Source: CAD feature listing. Evaluate the final solid. Frame: model axes, mm. Face numbers are marked on the shaded views. Give positions to 0.01 mm unless a question says otherwise; leave off trailing zeros. Loops run counter-clockwise (first coordinate to the right, second up) from the corner with the lowest first, then second, coordinate; pieces in that order, holes last. Notation, with made-up numbers: M 69,-17 L 89,-17 A13 ccw 89,-12 Z; hole C -26.5,0 d7. An arc over 180 degrees is marked long. Put each result on its own line as item: value. Start each with the question number.
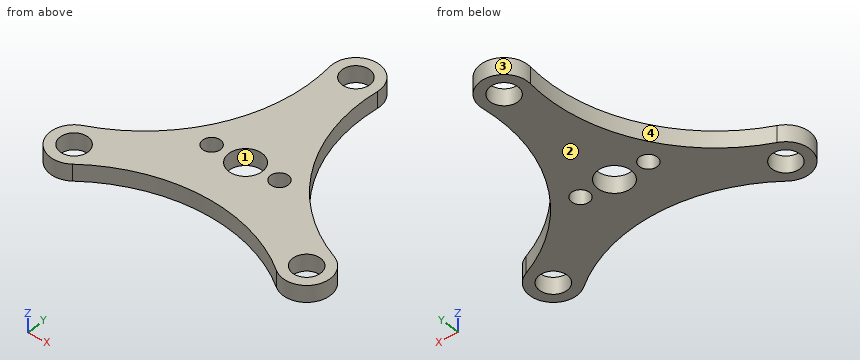
```python
from build123d import *

# Parameters (mm, degrees)
SKETCH_1_R      = 2.5
SKETCH_1_R_2    = 3
SKETCH_1_R_3    = 1.6
EXTRUDE_1_DEPTH = 3


with BuildPart() as part:
    # ｽｹｯﾁ1 → ﾎﾞｽ - 押し出し1 (new body)
    with BuildSketch(Plane.XY):
        with BuildLine():
            ThreePointArc((-22.235006429, -7.965532761), (-24.248711306, -14), (-18.01585694, -15.27331404))
            ThreePointArc((-18.01585694, -15.27331404), (0, -9.261413146), (18.01585694, -15.27331404))
            ThreePointArc((18.01585694, -15.27331404), (24.248711306, -14), (22.235006429, -7.965532761))
            ThreePointArc((22.235006429, -7.965532761), (8.020619059, 4.630706573), (4.219149489, 23.238846801))
            ThreePointArc((4.219149489, 23.238846801), (0, 28), (-4.219149489, 23.238846801))
            ThreePointArc((-4.219149489, 23.238846801), (-8.020619059, 4.630706573), (-22.235006429, -7.965532761))
        make_face()
        with Locations((0, 23.75)):
            Circle(SKETCH_1_R, mode=Mode.SUBTRACT)
        Circle(SKETCH_1_R_2, mode=Mode.SUBTRACT)
        with Locations((-6, 0)):
            Circle(SKETCH_1_R_3, mode=Mode.SUBTRACT)
        with Locations((6, 0)):
            Circle(SKETCH_1_R_3, mode=Mode.SUBTRACT)
        with Locations((20.56810334, -11.875)):
            Circle(SKETCH_1_R, mode=Mode.SUBTRACT)
        with Locations((-20.56810334, -11.875)):
            Circle(SKETCH_1_R, mode=Mode.SUBTRACT)
    extrude(amount=EXTRUDE_1_DEPTH)


solid = part.part
```
1. Pull-direction query (X, two-part tool) for the marked faces 1, 2, 3 and 4; classes: released by +X, released by -X, zero draft, split by the parting line, or undercut.
2. Section A-A, the plane x = 0. Output: boundary loops of the cut face in (y, z), plus the area to 3 significant figures.
3. Section C-C, the plane z = 1.3. Output: boundary loops of the cut face in (x, y) (3 decimals), plus the area to 3 significant figures.
4. Section D-D, the plane y = 0. Output: boundary loops of the cut face in (x, z), plus the area to 3 significant figures.
5. Ray query, line 1 (Y direction, x = 0, z = 2.3); line 2 (X direction, y = -14, z = 2.65); line 3 (Y direction, x = -22, z = 2.55). Return the intervals inside material, ascending.
6. Section B-B, the plane x = 6. Output: boundary loops of the cut face in (y, z), plus the area to 3 significant figures.
7. Contact query for flat-ended pins moving along their axis: pin 1 (1 mm diameter, centred on x = -1.5, z = 1.5, fed in from +Y); pin 2 (1.5 mm diameter, centred on x = 15, z = 1.5, fed in from -Y); pin 3 (1 mm diameter, centred on y = 17.5, z = 2, fed in from -X). Output: stop coordinate, or through.
Results found:
1. face 1: undercut
1. face 2: zero draft
1. face 3: split by the parting line
1. face 4: released by -X
2. outline: M -9.26,0 L -3,0 L -3,3 L -9.26,3 Z; M 3,0 L 21.25,0 L 21.25,3 L 3,3 Z; M 26.25,0 L 28,0 L 28,3 L 26.25,3 Z
2. area: 78.8 mm²
3. outline: M -22.235,-7.966 A4.25 ccw long -18.016,-15.273 A30 cw 18.016,-15.273 A4.25 ccw long 22.235,-7.966 A30 cw 4.219,23.239 A4.25 ccw long -4.219,23.239 A30 cw Z; hole C -20.568,-11.875 d5; hole C -6,0 d3.2; hole C 0,0 d6; hole C 0,23.75 d5; hole C 6,0 d3.2; hole C 20.568,-11.875 d5
3. area: 672 mm²
4. outline: M -11.32,0 L -7.6,0 L -7.6,3 L -11.32,3 Z; M -4.4,0 L -3,0 L -3,3 L -4.4,3 Z; M 3,0 L 4.4,0 L 4.4,3 L 3,3 Z; M 7.6,0 L 11.32,0 L 11.32,3 L 7.6,3 Z
4. area: 30.7 mm²
5. line 1: -9.26 to -3, 3 to 21.25, 26.25 to 28
5. line 2: -24.25 to -21.89, -19.25 to -16.18, 16.18 to 19.25, 21.89 to 24.25
5. line 3: -15.88 to -13.92, -9.83 to -7.86
6. outline: M -9.87,0 L -1.6,0 L -1.6,3 L -9.87,3 Z; M 1.6,0 L 8.86,0 L 8.86,3 L 1.6,3 Z
6. area: 46.6 mm²
7. pin 1: y = 27.88
7. pin 2: y = -13.73
7. pin 3: x = -4.12
